```python
from build123d import *

# Parameters (mm, degrees)
BOSS_EXTRUDE1_DEPTH = 20
SKETCH2_R           = 2.2
CUT_EXTRUDE1_DEPTH  = 3


with BuildPart() as part:
    # Sketch1 → Boss-Extrude1 (new body)
    with BuildSketch(Plane(origin=(0, 0, 0), x_dir=(1, 0, 0), z_dir=(0, 1, 0))):
        with BuildLine():
            Line((24.549928775, -5.633868186), (24.549928775, -1))
            Line((24.549928775, -1), (14.966629547, -1))
            ThreePointArc((14.966629547, -1), (-15, 0), (14.966629547, 1))
            Line((14.966629547, 1), (24.549928775, 1))
            Line((24.549928775, 1), (24.549928775, 9.723102863))
            Line((24.549928775, 9.723102863), (24.549928775, 23))
            Line((24.549928775, 23), (21.549928775, 23))
            Line((21.549928775, 23), (21.549928775, 4))
            Line((21.549928775, 4), (17.549928775, 4))
            ThreePointArc((17.549928775, 4), (-18, 0), (17.549928775, -4))
            Line((17.549928775, -4), (21.549928775, -4))
            Line((21.549928775, -4), (21.549928775, -23))
            Line((21.549928775, -23), (24.549928775, -23))
            Line((24.549928775, -23), (24.549928775, -5.633868186))
        make_face()
    extrude(amount=BOSS_EXTRUDE1_DEPTH)

    # Sketch2 → Cut-Extrude1 (cut)
    with BuildSketch(Plane(origin=(24.549928775, 0, 0), x_dir=(0, 0, -1), z_dir=(1, 0, 0))):
        with Locations((19, 10)):
            Circle(SKETCH2_R)
        with Locations((-19, 10)):
            Circle(SKETCH2_R)
    extrude(amount=-CUT_EXTRUDE1_DEPTH, mode=Mode.SUBTRACT)


solid = part.part
```
The model under review builds one solid part; all positions refer to its coordinate system, in mm. A direction names the side the tool comes from. Round coordinates to 2 decimals unless told otherwise and drop trailing zeros. Write each loop counter-clockwise with the first axis right and the second up, starting at its lowest first coordinate (ties: lowest second). Pieces come first, ordered by that corner, then holes. Notation, with made-up numbers: (63, 64.5) - (73, 64.5) arc R15 cw to (73, 69.5) - close; hole circle Ø3 at (12.5, 38.25). An arc over 180 degrees is marked (long way). Answer as CSV lines item,"result". Start each with the question number.
(1) For faces 4 (the flat face through (20, 10, -4)), 5 (the flat face through (24.55, 10, -12)), 6 (the flat face through (21.55, 10, 13)), 7 (the flat face through (20, 10, 1)), 8 (the cylindrical face through (23.07, 10.66, 16.9)), list the 3-axis set-ups (+Z, -Z, +X, -X, +Y, -Y) from which the entire face can be reached by the end or side of a thin tool; tool diameter is ignored.
(2) For pin 1 Ø2 at (x, y) = (20.5, 9) entering from -Z; pin 2 Ø1.2 at (x, y) = (20.5, 12) entering from +Z; pin 3 Ø4 at (y, z) = (9.5, 14) entering from -X, all flat-tipped, find the tip position at first contact; note any pin that passes through.
(3) We need section C-C on x = 2.5. State the section outline as (y, z) points, plus the area to 3 significant figures.
(4) To check wall thickness, follow line 1 (Z direction, x = 0, y = 5.75); line 2 (X direction, y = 11.5, z = -4.5); line 3 (X direction, y = 2, z = 12.5). State the ranges of each line that lie inside material, in increasing order.
(5) We need section B-B on y = 10. State the section outline as (x, z) points.
(6) We need section A-A on z = 19. State the section outline as (x, y) points.
(7) We need section D-D on z = -9. State the section outline as (x, y) points.
(8) Draft analysis for pull direction Y (two halves, no side actions). For faces 1 (the flat face through (16, 20, 2)), 2 (the cylindrical face through (23.07, 10.66, -21.1)), 3 (the cylindrical face through (-17.985, 9.86, -0.735)), state which applies: pulls with the +Y half, pulls with the -Y half, needs draft (parallel to the pull), parting line crosses it, or undercut.
Worked answers:
1,face 4,"-Z, +Y, -Y"
1,face 5,"+Z, -Z, +X, +Y, -Y"
1,face 6,"+Z, +Y, -Y"
1,face 7,"+X, +Y, -Y"
1,face 8,"+X"
2,pin 1,"z = -4"
2,pin 2,"z = 4"
2,pin 3,"x = -13.42"
3,outline,"(0, -17.83) - (20, -17.83) - (20, -14.79) - (0, -14.79) - close; (0, 14.79) - (20, 14.79) - (20, 17.83) - (0, 17.83) - close"
3,area,"121 mm²"
4,line 1,"-18 to -15, 15 to 18"
4,line 2,"-17.43 to -14.31, 14.31 to 17.43, 21.55 to 24.55"
4,line 3,"-12.95 to -8.29, 8.29 to 12.95, 21.55 to 24.55"
5,outline,"(14.97, -1) arc R15 cw (long way) to (14.97, 1) - (24.55, 1) - (24.55, 16.8) - (21.55, 16.8) - (21.55, 4) - (17.55, 4) arc R18 ccw (long way) to (17.55, -4) - (21.55, -4) - (21.55, -16.8) - (24.55, -16.8) - (24.55, -1) - close; (21.55, -23) - (24.55, -23) - (24.55, -21.2) - (21.55, -21.2) - close; (21.55, 21.2) - (24.55, 21.2) - (24.55, 23) - (21.55, 23) - close"
6,outline,"(21.55, 0) - (24.55, 0) - (24.55, 7.8) - (21.55, 7.8) - close; (21.55, 12.2) - (24.55, 12.2) - (24.55, 20) - (21.55, 20) - close"
7,outline,"(-15.59, 0) - (-12, 0) - (-12, 20) - (-15.59, 20) - close; (12, 0) - (15.59, 0) - (15.59, 20) - (12, 20) - close; (21.55, 0) - (24.55, 0) - (24.55, 20) - (21.55, 20) - close"
8,face 1,"pulls with the +Y half"
8,face 2,"undercut"
8,face 3,"needs draft"
